Verification items for the finished model (mm, model axes). Face numbers are marked on the shaded views. A direction names the side the tool comes from. Give positions to 0.01 mm unless a question says otherwise; leave off trailing zeros. Order: outer loops, then holes, each group sorted by start corner. A loop starts at its lowest first (then second) coordinate and runs counter-clockwise, first axis right, second up.
from build123d import *

# Parameters (mm, degrees)
SKETCH2_W           = 30
SKETCH2_H           = 40
BOSS_EXTRUDE2_DEPTH = 25
FILLET2_R           = 1
FILLET3_R           = 1
SHELL1_START        = 1.5
SHELL1_OUTLINE_W    = 37
SHELL1_OUTLINE_H    = 23.5
SHELL1_DEPTH        = 27
FILLET4_R           = 1
SKETCH5_W           = 3
SKETCH5_H           = 10
CUT_EXTRUDE1_DEPTH  = 56.901699437


# Read off the part's stored shape, not the designer's step: Shell1
with BuildPart() as part:
    # Sketch2 → Boss-Extrude2 (new body)
    with BuildSketch(Plane.XY):
        with Locations((15, 20)):
            Rectangle(SKETCH2_W, SKETCH2_H)
    extrude(amount=BOSS_EXTRUDE2_DEPTH)

    # Fillet2
    fillet2_edges = [part.edges().sort_by_distance(p)[0] for p in [
        (30, 20, 25),
        (15, 0, 25),
        (0, 20, 25),
        (15, 40, 25),
    ]]
    fillet(fillet2_edges, radius=FILLET2_R)

    # Fillet3
    # the kernel refuses this fillet: 1 mm, written as the material it takes off along each edge
    with BuildSketch(Plane(origin=(1, 39, 24), x_dir=(0, 1, 0), z_dir=(-1, 0, 0))) as fillet3_piece_1_section:
        Polygon((0, 0), (FILLET3_R, 0), (FILLET3_R, -FILLET3_R), (0, -FILLET3_R), align=None)
    fillet3_piece_1 = extrude(amount=FILLET3_R, mode=Mode.PRIVATE)
    fillet3_piece_1 = fillet3_piece_1 - Plane(origin=(1, 39, 24), x_dir=(0, -0.7071067811865475, -0.7071067811865475), z_dir=(-1, 0, 0)) * Sphere(FILLET3_R, mode=Mode.PRIVATE)
    add(fillet3_piece_1, mode=Mode.SUBTRACT)
    with BuildSketch(Plane(origin=(29, 39, 24), x_dir=(0, 1, 0), z_dir=(1, 0, 0))) as fillet3_piece_2_section:
        Polygon((0, 0), (FILLET3_R, 0), (FILLET3_R, FILLET3_R), (0, FILLET3_R), align=None)
    fillet3_piece_2 = extrude(amount=FILLET3_R, mode=Mode.PRIVATE)
    fillet3_piece_2 = fillet3_piece_2 - Plane(origin=(29, 39, 24), x_dir=(0, -0.7071067811865475, -0.7071067811865475), z_dir=(1, 0, 0)) * Sphere(FILLET3_R, mode=Mode.PRIVATE)
    add(fillet3_piece_2, mode=Mode.SUBTRACT)
    with BuildSketch(Plane(origin=(1, 1, 24), x_dir=(-1, 0, 0), z_dir=(0, -1, 0))) as fillet3_piece_3_section:
        Polygon((0, 0), (FILLET3_R, 0), (FILLET3_R, -FILLET3_R), (0, -FILLET3_R), align=None)
    fillet3_piece_3 = extrude(amount=FILLET3_R, mode=Mode.PRIVATE)
    fillet3_piece_3 = fillet3_piece_3 - Plane(origin=(1, 1, 24), x_dir=(0.7071067811865475, 0, -0.7071067811865475), z_dir=(0, -1, 0)) * Sphere(FILLET3_R, mode=Mode.PRIVATE)
    add(fillet3_piece_3, mode=Mode.SUBTRACT)
    with BuildSketch(Plane(origin=(29, 1, 24), x_dir=(1, 0, 0), z_dir=(0, -1, 0))) as fillet3_piece_4_section:
        Polygon((0, 0), (FILLET3_R, 0), (FILLET3_R, FILLET3_R), (0, FILLET3_R), align=None)
    fillet3_piece_4 = extrude(amount=FILLET3_R, mode=Mode.PRIVATE)
    fillet3_piece_4 = fillet3_piece_4 - Plane(origin=(29, 1, 24), x_dir=(-0.7071067811865475, 0, -0.7071067811865475), z_dir=(0, -1, 0)) * Sphere(FILLET3_R, mode=Mode.PRIVATE)
    add(fillet3_piece_4, mode=Mode.SUBTRACT)
    with BuildSketch(Plane(origin=(30, 0, -2.5), x_dir=(-1, 0, 0), z_dir=(0, 0, 1)), Plane(origin=(30, 40, -2.5), x_dir=(0, -1, 0), z_dir=(0, 0, 1))) as fillet3_piece_5:
        with BuildLine():
            CenterArc((FILLET3_R, -FILLET3_R), FILLET3_R, 90, 90)
            Line((0, -FILLET3_R), (0, 0))
            Line((0, 0), (FILLET3_R, 0))
        make_face()
    extrude(amount=26.5, mode=Mode.SUBTRACT)
    with BuildSketch(Plane(origin=(0, 0, -2.5), x_dir=(1, 0, 0), z_dir=(0, 0, 1)), Plane(origin=(0, 40, -2.5), x_dir=(0, -1, 0), z_dir=(0, 0, 1))) as fillet3_piece_6:
        with BuildLine():
            CenterArc((FILLET3_R, FILLET3_R), FILLET3_R, 180, 90)
            Line((0, FILLET3_R), (0, 0))
            Line((0, 0), (FILLET3_R, 0))
        make_face()
    extrude(amount=26.5, mode=Mode.SUBTRACT)

    # Shell1 outline → Shell1 (cut)
    with BuildSketch(Plane.YZ.offset(SHELL1_START)):
        with Locations((20, 11.75)):
            Rectangle(SHELL1_OUTLINE_W, SHELL1_OUTLINE_H)
    extrude(amount=SHELL1_DEPTH, mode=Mode.SUBTRACT)

    # Fillet4
    fillet4_edges = [part.edges().sort_by_distance(p)[0] for p in [
        (28.5, 20, 23.5),
        (1.5, 20, 23.5),
        (15, 1.5, 23.5),
        (15, 38.5, 23.5),
    ]]
    fillet(fillet4_edges, radius=FILLET4_R)

    # Sketch5 → Cut-Extrude1 (cut, through all)
    with BuildSketch(Plane.XY.offset(25)):
        with Locations((21.5, 25)):
            Rectangle(SKETCH5_W, SKETCH5_H)
    extrude(amount=-CUT_EXTRUDE1_DEPTH, mode=Mode.SUBTRACT)


solid = part.part
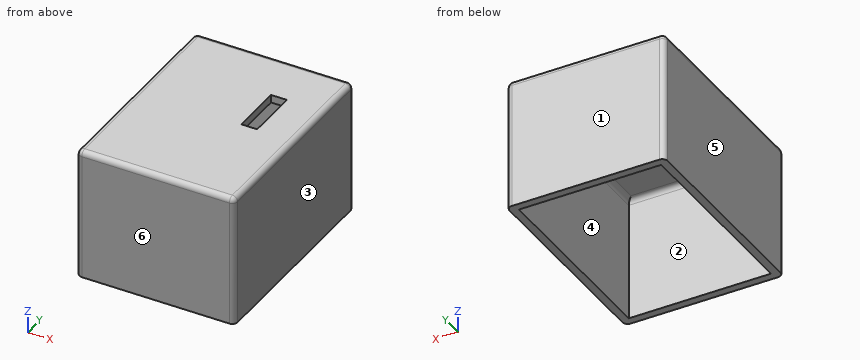
(1) Section check C-C, the plane x = 15. Enter the section's corners in (y, z), then the cut area to 4 significant figures.
Solved:
outline: (0, 0) - (1.5, 0) - (1.5, 22.5) arc R1 cw to (2.5, 23.5) - (37.5, 23.5) arc R1 cw to (38.5, 22.5) - (38.5, 0) - (40, 0) - (40, 24) arc R1 ccw to (39, 25) - (1, 25) arc R1 ccw to (0, 24) - close
area: 130.5 mm2
(2) Release check for a two-part mould opening along X. For the marked faces 3, 4, 5 and 6 record: pulls with the +X half, pulls with the -X half, needs draft (parallel to the pull), parting line crosses it, or undercut.
Solved:
face 3: pulls with the +X half
face 4: undercut
face 5: pulls with the -X half
face 6: needs draft
(3) Go/stop test with flat-tipped pins: pin 1 (4 mm diameter, centred on x = 18, y = 29.5, fed in from -Z); pin 2 (1.2 mm diameter, centred on y = 25, z = 24.5, fed in from -X). Record where each tip stops, or that it passes through.
Solved:
pin 1: stops at z = 23.5
pin 2: stops at x = 0
(4) Section check A-A, the plane y = 26.5. Enter the section's corners in (x, z).
Solved:
outline: (0, 0) - (1.5, 0) - (1.5, 22.5) arc R1 cw to (2.5, 23.5) - (20, 23.5) - (20, 25) - (1, 25) arc R1 ccw to (0, 24) - close; (23, 23.5) - (27.5, 23.5) arc R1 cw to (28.5, 22.5) - (28.5, 0) - (30, 0) - (30, 24) arc R1 ccw to (29, 25) - (23, 25) - close
(5) Scan lines: line 1 (X direction, y = 19.5, z = 9); line 2 (Y direction, x = 9, z = 14); line 3 (Z direction, x = 9, y = 26). Record each from-to range of solid material in increasing order.
Solved:
line 1: x = 0 to 1.5, 28.5 to 30
line 2: y = 0 to 1.5, 38.5 to 40
line 3: z = 23.5 to 25
(6) Section check D-D, the plane y = 4. Enter the section's corners in (x, z), then the cut area to 4 significant figures.
Solved:
outline: (0, 0) - (1.5, 0) - (1.5, 22.5) arc R1 cw to (2.5, 23.5) - (27.5, 23.5) arc R1 cw to (28.5, 22.5) - (28.5, 0) - (30, 0) - (30, 24) arc R1 ccw to (29, 25) - (1, 25) arc R1 ccw to (0, 24) - close
area: 115.5 mm2
(7) Set-up check for the marked faces 1 and 2: record each of +Z, -Z, +X, -X, +Y, -Y from which the full face is reachable in a straight line by a thin tool's end or side.
Solved:
face 1: +Z, -Z, +X, -X, +Y
face 2: -Z
(8) Section check B-B, the plane z = 13.25. Enter the section's corners in (x, y), then the cut area to 3 significant figures.
Solved:
outline: (0, 1) arc R1 ccw to (1, 0) - (29, 0) arc R1 ccw to (30, 1) - (30, 39) arc R1 ccw to (29, 40) - (1, 40) arc R1 ccw to (0, 39) - close; hole (1.5, 1.5) - (28.5, 1.5) - (28.5, 38.5) - (1.5, 38.5) - close
area: 200 mm2
